Input: part model. Units: mm. Frame: model coordinates. A direction names the side the tool comes from. Coordinates: 2 decimals unless noted, no trailing zeros. Loops run counter-clockwise (first coordinate to the right, second up) from the corner with the lowest first, then second, coordinate; pieces in that order, holes last. Notation, with made-up numbers: (29, 71.25) -> (39, 71.25) arc R14 cw to (39, 86.25) -> close; hole circle Ø2 at (14.5, 31). An arc over 180 degrees is marked (long way). Answer as a JSON object with one key per item and string values.
from build123d import *

# Parameters (mm, degrees)
F0_W      = 16.764
F0_H      = 17.907
F0_W_2    = 12.7
F0_H_2    = 12.7
F1_DEPTH  = 19.05
F2_W      = 21.1890064
F2_H      = 17.8200355506
F3_DEPTH  = 25.4
F4_R      = 6.35
F5_DEPTH  = 76.2
F7_DEPTH  = 19.05
F8_DEPTH  = 79.375
F9_R      = 3.175
F10_R     = 1.016
F12_DEPTH = 25.4
F13_W     = 9.1727420804
F13_H     = 4.4667599723
F13_W_2   = 3.1133545563
F13_H_2   = 8.6221548263
F14_DEPTH = 6.35


with BuildPart() as f1:
    # F0 (on Front) → F1 (new body)
    with BuildSketch(Plane.XZ):
        with Locations((8.382, 8.9535)):
            Rectangle(F0_W, F0_H)
        with Locations((8.382, 9.525)):
            Rectangle(F0_W_2, F0_H_2, mode=Mode.SUBTRACT)
    extrude(amount=F1_DEPTH)

    # F2 (on Front) → F3 (cut)
    with BuildSketch(Plane.XZ):
        with Locations((15.1665032, 14.6250177753)):
            Rectangle(F2_W, F2_H)
    extrude(amount=F3_DEPTH, mode=Mode.SUBTRACT)

    # F4 (on face) → F5 (join)
    with BuildSketch(Plane(origin=(0, 0, 0), x_dir=(1, 0, 0), z_dir=(0, 0, -1))):
        with Locations((8.382, 9.525)):
            Circle(F4_R)
    extrude(amount=F5_DEPTH)

    # F6 (on Front) → F7 (join)
    with BuildSketch(Plane.XZ):
        with BuildLine():
            Line((46.482, -88.5501227317), (46.482, -81.894013743))
            ThreePointArc((46.482, -81.894013743), (8.382, -76.2), (-29.718, -81.894013743))
            Line((-29.718, -81.894013743), (-29.718, -88.5501227317))
            ThreePointArc((-29.718, -88.5501227317), (8.382, -82.55), (46.482, -88.5501227317))
        make_face()
    extrude(amount=F7_DEPTH)

    # F4 (on face) → F8 (join)
    with BuildSketch(Plane(origin=(0, 0, 0), x_dir=(1, 0, 0), z_dir=(0, 0, -1))):
        with Locations((8.382, 9.525)):
            Circle(F4_R)
    extrude(amount=F8_DEPTH)

    # F9
    f9_edges = [f1.edges().sort_by_distance(p)[0] for p in [
        (8.382, -19.05, -82.55),
        (46.482, -9.525, -88.550123),
        (46.482, -19.05, -85.222068),
        (-29.718, -19.05, -85.222068),
        (-29.718, 0, -85.222068),
        (8.382, 0, -82.55),
        (-29.718, -9.525, -88.550123),
        (46.482, 0, -85.222068),
    ]]
    fillet(f9_edges, radius=F9_R)

    # F10
    f10_edges = [f1.edges().sort_by_distance(p)[0] for p in [
        (4.572, -9.525, 15.875),
        (14.732, -9.525, 5.715),
    ]]
    fillet(f10_edges, radius=F10_R)

    # F11 (on Right) → F12 (cut)
    with BuildSketch(Plane.YZ):
        Polygon((-9.525, -1.4437012938), (-12.7, -1.4437012938), (-12.7, -3.9837012938), (-6.35, -3.9837012938), (-6.35, -1.4437012938), align=None)
    extrude(amount=F12_DEPTH, mode=Mode.SUBTRACT)

    # F13 (on face) → F14 (cut, through all)
    with BuildSketch(Plane.XZ.offset(6.35)):
        with Locations((3.6581899913, 18.1083799861)):
            Rectangle(F13_W, F13_H)
        with Locations((16.2886772781, 2.7195581933)):
            Rectangle(F13_W_2, F13_H_2)
    extrude(amount=F14_DEPTH, mode=Mode.SUBTRACT)


solid = f1.part
1. Mould query, pull axis Z, two halves, no side actions, for faces 1 (the face through (8.9, -3, -76.2)), 2 (the face through (-28.422, -9.614, -86.825)), 3 (the face through (8, -6.35, -3)), 4 (the face through (2, -6.35, 17)). Classes: pulls with the +Z half, pulls with the -Z half, needs draft (parallel to the pull), parting line crosses it, or undercut.
Reply:
{"face 1": "undercut", "face 2": "pulls with the -Z half", "face 3": "undercut", "face 4": "needs draft"}
2. Section query C-C (z = -73). Return loops of the section in (x, y) (3 decimals).
Reply:
{"outline": "circle Ø12.7 at (8.382, -9.525)"}
3. Line query: line 1 along X through (y, z) = (-10, -44.5); line 2 along X through (y, z) = (-2.25, 8); line 3 along Z through (x, y) = (4.5, -7.25) (3 decimals). Output: solid intervals per line, ascending.
Reply:
{"line 1": "x = 2.05 to 14.71", "line 2": "x = 0 to 2.03", "line 3": "z = -82.611 to -3.984, -1.444 to 3.175"}
4. Pin query (flat end, axial travel): P1, Ø10, axis at x = 11, y = -7, coming from the +Z side (3 decimals); P2, Ø0.8, axis at y = -15.5, z = 17.5, coming from the +X side; P3, Ø1.7, axis at x = 2.5, y = -2.5, coming from the -Z side. Return the tip coordinate at first contact, or that it passes through.
Reply:
{"P1": "stops at z = 5.715", "P2": "stops at x = 4.57", "P3": "stops at z = -82.72"}
5. Access query for faces 5 (the face through (16.764, -3, 3)), 6 (the face through (2.032, -9, 9)), 7 (the face through (8, -10, -3.984)), 8 (the face through (1, -9, 15.875)). Directions: +Z, -Z, +X, -X, +Y, -Y. A direction counts if a zero-diameter tool reaches every point of the face in a straight line with its end or side. Return the directions, or none.
Reply:
{"face 5": "+Z, +X, +Y, -Y", "face 6": "+Y, -Y", "face 7": "+X, -X", "face 8": "+Z, +X, -X"}
6. Section query A-A (y = -7.75). Return loops of the section in (x, z) (3 decimals).
Reply:
{"outline": "(-29.718, -84.266) arc R3.175 ccw to (-25.671, -87.319) arc R123.965 cw to (42.435, -87.319) arc R3.175 ccw to (46.482, -84.266) -> (46.482, -81.894) arc R130.315 ccw to (14.479, -76.343) -> (14.479, -3.984) -> (2.285, -3.984) -> (2.285, -76.343) arc R130.315 ccw to (-29.718, -81.894) -> close; (0, 0) -> (2.285, 0) -> (2.285, -1.444) -> (14.479, -1.444) -> (14.479, 0) -> (14.732, 0) -> (14.732, 3.175) -> (2.032, 3.175) -> (2.032, 15.875) -> (0, 15.875) -> close"}
7. Section query B-B (y = -14.75). Return loops of the section in (x, z) (3 decimals), plus the area to 3 significant figures.
Reply:
{"outline": "(-29.718, -84.266) arc R3.175 ccw to (-25.671, -87.319) arc R123.965 cw to (42.435, -87.319) arc R3.175 ccw to (46.482, -84.266) -> (46.482, -81.894) arc R130.315 ccw to (11.991, -76.25) -> (11.991, 0) -> (16.764, 0) -> (16.764, 5.715) -> (15.748, 5.715) arc R1.016 ccw to (14.732, 4.699) -> (14.732, 3.175) -> (2.032, 3.175) -> (2.032, 15.875) -> (3.556, 15.875) arc R1.016 ccw to (4.572, 16.891) -> (4.572, 17.907) -> (0, 17.907) -> (0, 0) -> (4.773, 0) -> (4.773, -76.25) arc R130.315 ccw to (-29.718, -81.894) -> close", "area": "1,130 mm2"}
